from build123d import *

# Parameters (mm, degrees)
TABAN_FLAN_1_DEPTH = 2550


# Sheet-metal steps are written as plain solids
with BuildPart() as part:
    # Çizim1 → Taban-Flanş1 (new body)
    with BuildSketch(Plane.XY):
        with BuildLine():
            Line((0, 0), (0, -395.029437252))
            ThreePointArc((0, -395.029437252), (0.91344561, -399.62163844), (3.514718626, -403.514718626))
            Line((3.514718626, -403.514718626), (196.485281374, -596.485281374))
            ThreePointArc((196.485281374, -596.485281374), (200.37836156, -599.08655439), (204.970562748, -600))
            Line((204.970562748, -600), (760, -600))
            Line((760, -600), (760, -594))
            Line((760, -594), (204.970562748, -594))
            ThreePointArc((204.970562748, -594), (202.674462154, -593.543277195), (200.727922061, -592.242640687))
            Line((200.727922061, -592.242640687), (7.757359313, -399.272077939))
            ThreePointArc((7.757359313, -399.272077939), (6.456722805, -397.325537846), (6, -395.029437252))
            Line((6, -395.029437252), (6, 0))
            Line((6, 0), (0, 0))
        make_face()
    extrude(amount=-TABAN_FLAN_1_DEPTH)


solid = part.part
Geometry: final body of the model. Coordinates: model frame, mm. A direction names the side the tool comes from. Give positions to 0.01 mm unless a question says otherwise; leave off trailing zeros. Write each loop counter-clockwise with the first axis right and the second up, starting at its lowest first coordinate (ties: lowest second). Pieces come first, ordered by that corner, then holes. Notation, with made-up numbers: M 80.5,6.5 L 88.5,6.5 A22 cw 88.5,41.5 Z; hole C 44.25,27 d5. An arc over 180 degrees is marked long. Answer in a Markdown table with one row per item. Add a question column.
(1) Section A-A on z = -1226. Return loops of the section in (x, y).
(2) Section B-B on x = 380.5. Return loops of the section in (y, z).
(3) Reachability of faces 1 (the flat face through (486, -594, -1257)), 2 (the flat face through (99, -499, -1257)) from +Z, -Z, +X, -X, +Y, -Y: full face, straight path, thin tool, end or side. Return the list, or none.
(4) Section C-C on y = -119.5. Return loops of the section in (x, z).
(5) Ray query, line 1 (X direction, y = -104.5, z = -2024); line 2 (Y direction, x = 249, z = -1577); line 3 (Y direction, x = 92, z = -218). Return the intervals inside material, ascending.
(6) First-contact query: pin 1 (6 mm diameter, centred on x = 223, z = -338, fed in from +Y); pin 2 (1.5 mm diameter, centred on y = -446, z = -370, fed in from -X). Flat tips, straight axial feed; report the tip coordinate or a pass-through.
Result set:
| question | item | result |
|---|---|---|
| 1 | outline | M 0,-395.03 A12 ccw 3.51,-403.51 L 196.49,-596.49 A12 ccw 204.97,-600 L 760,-600 L 760,-594 L 204.97,-594 A6 cw 200.73,-592.24 L 7.76,-399.27 A6 cw 6,-395.03 L 6,0 L 0,0 Z |
| 2 | outline | M -600,-2550 L -594,-2550 L -594,0 L -600,0 Z |
| 3 | face 1 | +Z, -Z, +X, +Y |
| 3 | face 2 | +Z, -Z, -X, -Y |
| 4 | outline | M 0,-2550 L 6,-2550 L 6,0 L 0,0 Z |
| 5 | line 1 | x = 0 to 6 |
| 5 | line 2 | y = -600 to -594 |
| 5 | line 3 | y = -492 to -483.51 |
| 6 | pin 1 | stops at y = -594 |
| 6 | pin 2 | stops at x = 45.25 |
